Check sheet for the drawn part. Datum: minimum x, y, z corner. Units: mm. Give positions to 0.01 mm unless a question says otherwise; leave off trailing zeros. Loops run counter-clockwise (first coordinate to the right, second up) from the corner with the lowest first, then second, coordinate; pieces in that order, holes last. Notation, with made-up numbers: (5, 10.25) - (42, 10.25) arc R8 cw to (42, 25.25) - close; hole circle Ø4 at (6, -12). An arc over 180 degrees is marked (long way). Use one line per item in the form item = value.
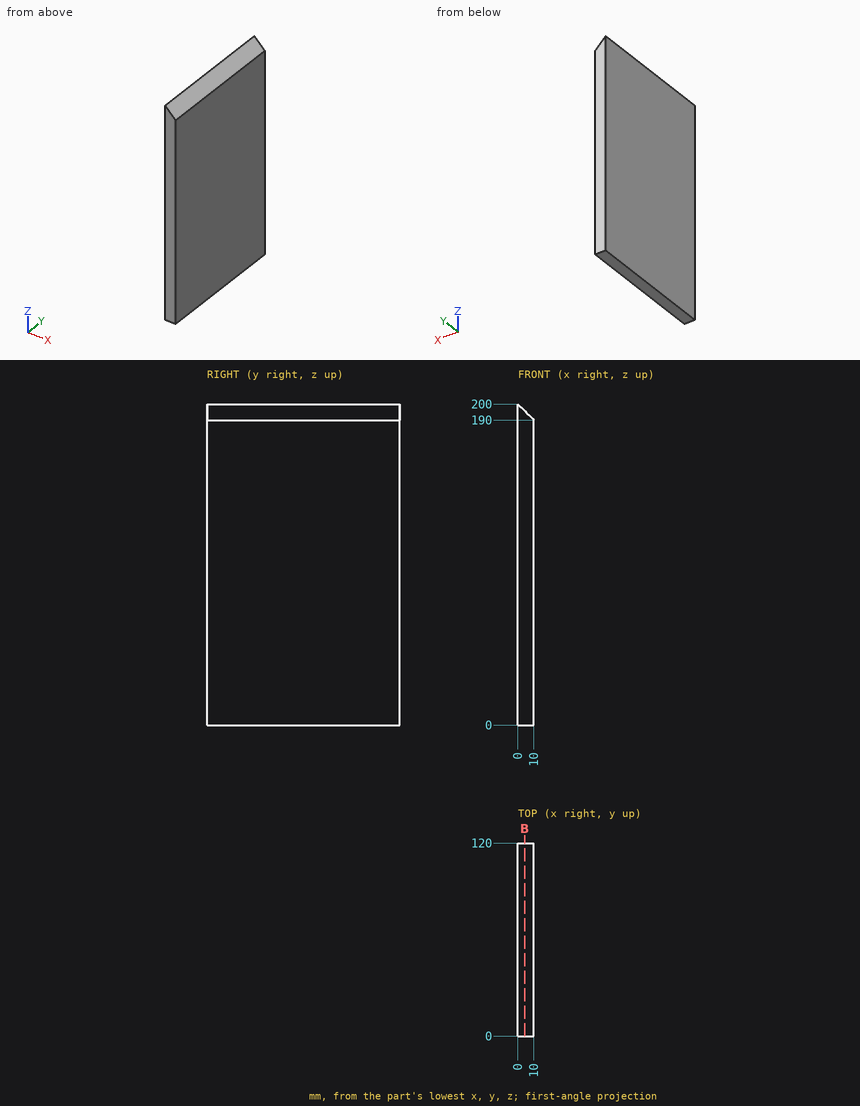
1. Scan lines: probe 1 along Z at (x, y) = (7.75, 55.5); probe 2 along Z at (x, y) = (6, 68.5); probe 3 along X at (y, z) = (79, 191.5). Record each from-to range of solid material in increasing order.
Result set:
probe_1 = 0 to 192.25
probe_2 = 0 to 194
probe_3 = 0 to 8.5
2. Section check B-B, the plane x = 4.25. Record the cut outline in (y, z), then the cut area to 3 significant figures.
Result set:
outline = (0, 0) - (120, 0) - (120, 195.75) - (0, 195.75) - close
area = 23,500 mm²
3. Depth check by flat-ended pin: pin 1 Ø1.5 at (x, y) = (7, 12.5) entering from +Z. Enter the tip coordinate at first touch or a pass-through.
Result set:
pin_1 = 193.75
